from build123d import *

# Parameters (mm, degrees)
BOSS_EXTRUDE2_DEPTH = 5
EXTRUDE_1_DEPTH     = 10


with BuildPart() as part:
    # Sketch3 → Boss-Extrude2 (new body)
    with BuildSketch(Plane.XY):
        with BuildLine():
            Line((-150.5, 80.5), (150.5, 80.5))
            ThreePointArc((150.5, 80.5), (157.571067812, 77.571067812), (160.5, 70.5))
            Line((160.5, 70.5), (160.5, -70.5))
            ThreePointArc((160.5, -70.5), (157.571067812, -77.571067812), (150.5, -80.5))
            Line((150.5, -80.5), (-150.5, -80.5))
            ThreePointArc((-150.5, -80.5), (-157.571067812, -77.571067812), (-160.5, -70.5))
            Line((-160.5, -70.5), (-160.5, 70.5))
            ThreePointArc((-160.5, 70.5), (-157.571067812, 77.571067812), (-150.5, 80.5))
        make_face()
    extrude(amount=-BOSS_EXTRUDE2_DEPTH)

    # Эскиз1 → Бобышка-Вытянуть1 (add)
    with BuildSketch(Plane(origin=(0, 0, 0), x_dir=(-1, 0, 0), z_dir=(0, 0, -1))):
        with BuildLine():
            Line((-150.5, -78.5), (150.5, -78.5))
            ThreePointArc((150.5, -78.5), (156.156854249, -76.156854249), (158.5, -70.5))
            Line((158.5, -70.5), (158.5, 70.5))
            ThreePointArc((158.5, 70.5), (156.156854249, 76.156854249), (150.5, 78.5))
            Line((150.5, 78.5), (-150.5, 78.5))
            ThreePointArc((-150.5, 78.5), (-156.156854249, 76.156854249), (-158.5, 70.5))
            Line((-158.5, 70.5), (-158.5, -70.5))
            ThreePointArc((-158.5, -70.5), (-156.156854249, -76.156854249), (-150.5, -78.5))
        make_face()
    extrude(amount=-EXTRUDE_1_DEPTH)


solid = part.part
For this review, take the finished solid that the model builds, in its own axes (mm). A direction names the side the tool comes from. Round coordinates to 2 decimals unless told otherwise and drop trailing zeros. Write each loop counter-clockwise with the first axis right and the second up, starting at its lowest first coordinate (ties: lowest second). Pieces come first, ordered by that corner, then holes. Notation, with made-up numbers: (76.25, 76) -> (106.25, 76) arc R9 cw to (106.25, 82) -> close; hole circle Ø5 at (-18.5, 57). An arc over 180 degrees is marked (long way). Use CSV: the item, a comma, the result in double quotes.
(1) For faces 1 (the face through (156.094, 76.219, 4.93)), 2 (the face through (-2, 78.5, 5)), 3 (the face through (-158.5, -1, 5)), 4 (the face through (158.5, 1, 5)), list the 3-axis set-ups (+Z, -Z, +X, -X, +Y, -Y) from which the entire face can be reached by the end or side of a thin tool; tool diameter is ignored.
Computed values:
face 1,"+Z, +X, +Y"
face 2,"+Z, +X, -X, +Y"
face 3,"+Z, -X, +Y, -Y"
face 4,"+Z, +X, +Y, -Y"
(2) Consider section A-A, the plane x = -69.5. Give the boundary of the cut face in (y, z).
Computed values:
outline,"(-80.5, -5) -> (80.5, -5) -> (80.5, 0) -> (78.5, 0) -> (78.5, 10) -> (-78.5, 10) -> (-78.5, 0) -> (-80.5, 0) -> close"
(3) Consider section B-B, the plane z = 3.5. Give the boundary of the cut face in (x, y), plus the area to 3 significant figures.
Computed values:
outline,"(-158.5, -70.5) arc R8 ccw to (-150.5, -78.5) -> (150.5, -78.5) arc R8 ccw to (158.5, -70.5) -> (158.5, 70.5) arc R8 ccw to (150.5, 78.5) -> (-150.5, 78.5) arc R8 ccw to (-158.5, 70.5) -> close"
area,"49,700 mm²"
(4) To check wall thickness, follow L1, parallel to X at y = 60, z = 3.5; L2, parallel to Y at x = -46, z = 0.25; L3, parallel to X at y = -71, z = -2.25. State the ranges of each line that lie inside material, in increasing order. Write a range as [from, to].
Computed values:
L1,"[-158.5, 158.5]"
L2,"[-78.5, 78.5]"
L3,"[-160.49, 160.49]"
(5) Clearance check with flat-ended pins moving along their axes: P1, Ø1.5, axis at x = 45, z = 1.5, coming from the -Y side; P2, Ø5, axis at y = -25.5, z = 4.5, coming from the -X side; P3, Ø3, axis at y = 10, z = 5.5, coming from the +X side. State where each tip first meets the part, or that it passes through.
Computed values:
P1,"y = -78.5"
P2,"x = -158.5"
P3,"x = 158.5"
